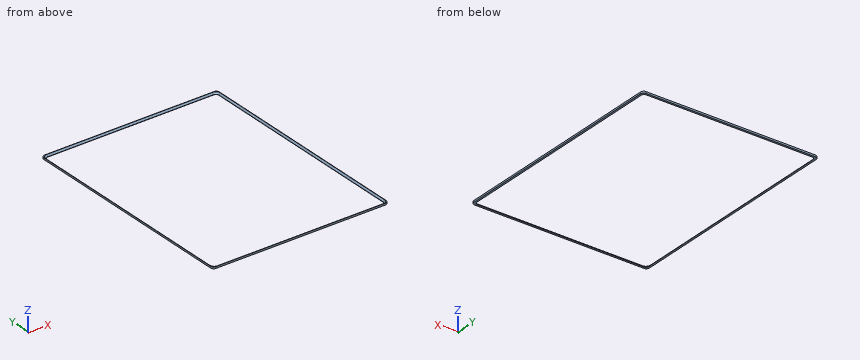
```python
from build123d import *

# Parameters (mm, degrees)
SKETCH_W     = 174
SKETCH_H     = 224
SKETCH_W_2   = 170.4
SKETCH_H_2   = 220.4
PAD_DEPTH    = 1.7
FILLET_R     = 3
CHAMFER_SIZE = 1.4


with BuildPart() as part:
    # Sketch → Pad (new body)
    with BuildSketch(Plane.XY):
        Rectangle(SKETCH_W, SKETCH_H)
        Rectangle(SKETCH_W_2, SKETCH_H_2, mode=Mode.SUBTRACT)
    extrude(amount=PAD_DEPTH)

    # Fillet
    fillet_edges = [part.edges().sort_by_distance(p)[0] for p in [
        (-85.2, -110.2, 0.85),
        (-87, -112, 0.85),
        (87, -112, 0.85),
        (85.2, -110.2, 0.85),
        (87, 112, 0.85),
        (85.2, 110.2, 0.85),
        (-85.2, 110.2, 0.85),
        (-87, 112, 0.85),
    ]]
    fillet(fillet_edges, radius=FILLET_R)

    # Chamfer
    chamfer_edges = [part.edges().sort_by_distance(p)[0] for p in [
        (-84.32132, -109.32132, 1.7),
    ]]
    chamfer(chamfer_edges, length=CHAMFER_SIZE)


solid = part.part
```
Input: part model. Units: mm. Frame: model coordinates. Give positions to 0.01 mm unless a question says otherwise; leave off trailing zeros. Order: outer loops, then holes, each group sorted by start corner. A loop starts at its lowest first (then second) coordinate and runs counter-clockwise, first axis right, second up. Notation, with made-up numbers: (89, -1) - (127, -1) arc R26 cw to (127, 17) - close; hole circle Ø9 at (32.25, -5.75). An arc over 180 degrees is marked (long way). One line per item, written item: value.
1. Line query: probe 1 along Y at (x, z) = (22, 0.1); probe 2 along Y at (x, z) = (-17.5, 1.65); probe 3 along X at (y, z) = (-83, 0.1). Output: solid intervals per line, ascending.
Determined:
probe 1: -112 to -110.2, 110.2 to 112
probe 2: -112 to -111.55, 111.55 to 112
probe 3: -87 to -85.2, 85.2 to 87
2. Cut plane B-B, the plane z = 1.25. Output: boundary loops of the cut face in (x, y), and give its area (3 significant figures).
Determined:
outline: (-87, -109) arc R3 ccw to (-84, -112) - (84, -112) arc R3 ccw to (87, -109) - (87, 109) arc R3 ccw to (84, 112) - (-84, 112) arc R3 ccw to (-87, 109) - close; hole (-86.15, -107.2) arc R3.95 ccw to (-82.2, -111.15) - (82.2, -111.15) arc R3.95 ccw to (86.15, -107.2) - (86.15, 107.2) arc R3.95 ccw to (82.2, 111.15) - (-82.2, 111.15) arc R3.95 ccw to (-86.15, 107.2) - close
area: 679 mm2
3. Cut plane C-C, the plane y = 0.5. Output: boundary loops of the cut face in (x, z).
Determined:
outline: (-87, 0) - (-85.2, 0) - (-85.2, 0.3) - (-86.6, 1.7) - (-87, 1.7) - close; (85.2, 0) - (87, 0) - (87, 1.7) - (86.6, 1.7) - (85.2, 0.3) - close
4. Cut plane A-A, the plane x = -36. Output: boundary loops of the cut face in (y, z).
Determined:
outline: (-112, 0) - (-110.2, 0) - (-110.2, 0.3) - (-111.6, 1.7) - (-112, 1.7) - close; (110.2, 0) - (112, 0) - (112, 1.7) - (111.6, 1.7) - (110.2, 0.3) - close
